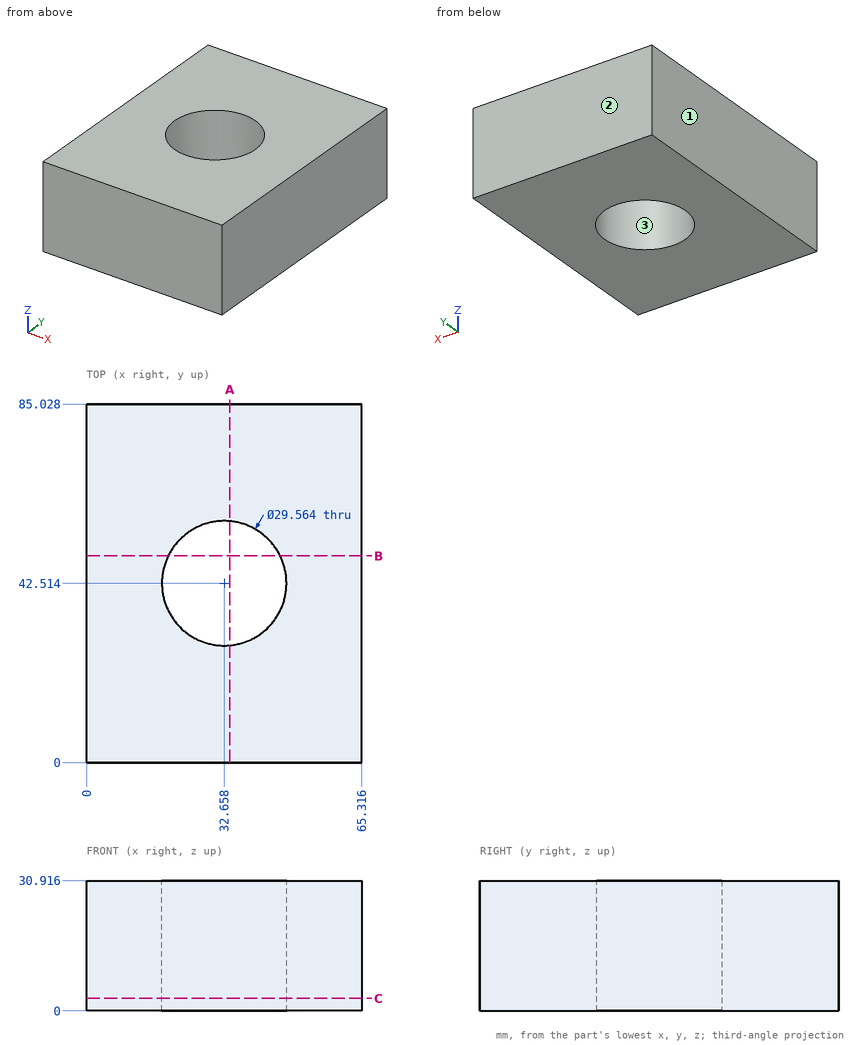
For this review, use the dimensioned drawing (mm, ordinates from the lowest corner) and the shaded views. Give positions to 0.01 mm unless a question says otherwise; leave off trailing zeros. Order: outer loops, then holes, each group sorted by start corner. A loop starts at its lowest first (then second) coordinate and runs counter-clockwise, first axis right, second up. Notation, with made-up numbers: (63.25, 75.25) - (101.25, 75.25) arc R22 ccw to (101.25, 112.25) - close; hole circle Ø6 at (17.25, 26). An arc over 180 degrees is marked (long way). Write item = value, one per line. Start each with the question number.
Q1. We need section B-B on y = 49. State the section outline as (x, z) points (1 decimal), plus the area to 3 significant figures.
Q2. We need section A-A on x = 34. State the section outline as (y, z) points (1 decimal).
Q3. We need section C-C on z = 3. State the section outline as (x, y) points (1 decimal).
Q4. Mouldability with a two-part tool opening along Y and no side actions: class the marked faces 1, 2 and 3 as released by +Y, released by -Y, zero draft, split by the parting line, or undercut.
Q5. To check wall thickness, follow L1, parallel to X at y = 47, z = 2 (1 decimal); L2, parallel to X at y = 54, z = 23 (1 decimal); L3, parallel to Y at x = 40, z = 18 (1 decimal). State the ranges of each line that lie inside material, in increasing order. Write a range as from..to.
Working result:
q1.outline = (0, 0) - (19.4, 0) - (19.4, 30.9) - (0, 30.9) - close; (45.9, 0) - (65.3, 0) - (65.3, 30.9) - (45.9, 30.9) - close
q1.area = 1,200 mm²
q2.outline = (0, 0) - (27.8, 0) - (27.8, 30.9) - (0, 30.9) - close; (57.2, 0) - (85, 0) - (85, 30.9) - (57.2, 30.9) - close
q3.outline = (0, 0) - (65.3, 0) - (65.3, 85) - (0, 85) - close; hole circle Ø29.6 at (32.7, 42.5)
q4.face_1 = zero draft
q4.face_2 = released by +Y
q4.face_3 = undercut
q5.L1 = 0..18.6, 46.7..65.3
q5.L2 = 0..23.4, 42..65.3
q5.L3 = 0..29.7, 55.3..85
